Check sheet for the modelled part. Datum: model origin and axes. Units: mm. Face numbers are marked on the shaded views. Coordinates: 2 decimals unless noted, no trailing zeros. Answer as CSV lines item,"result". Start each with the question number.
1) Material ranges on L1, parallel to X at y = -4, z = 5.5; L2, parallel to X at y = -12, z = 3.5; L3, parallel to X at y = 8.5, z = 1.75, recorded low to high. Write a range as [from, to].
2) Section check A-A (z = 5.75). State how many separate pieces and enclosed holes the cut face has, and give its area (3 significant figures).
3) Draft check along X on the marked faces 1, 2 and 3. Enter one of: +X half, -X half, draft (parallel to the pull), parting line (faces both ways), or undercut.
4) Go/stop test with flat-tipped pins: pin 1 Ø3 at (x, y) = (0, -21) entering from +Z; pin 2 Ø4.5 at (x, y) = (0, 21) entering from -Z; pin 3 Ø1.5 at (y, z) = (-12, 2.5) entering from +X; pin 4 Ø1 at (x, z) = (-8.5, 2.5) entering from -Y. Record where each tip stops, or that it passes through.
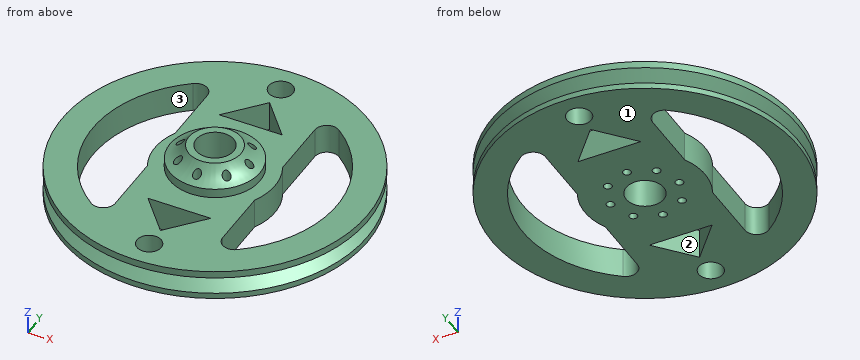
from build123d import *

# Parameters (mm, degrees)
F0_R      = 25.4
F0_R_2    = 3.125
F1_DEPTH  = 5
F2_R      = 7.5
F2_R_2    = 3.125
F3_DEPTH  = 4
F4_R      = 6.096
F6_R      = 2.020962
F7_DEPTH  = 5.001
F10_R     = 0.662213
F11_DEPTH = 9.001


with BuildPart() as f1:
    # F0 (on Top) → F1 (new body)
    with BuildSketch(Plane.XY):
        Circle(F0_R)
        with BuildLine():
            Line((-8.950036, 14.687379), (-8.950036, 4.46059))
            ThreePointArc((-8.950036, 4.46059), (-10, 0), (-8.950036, -4.46059))
            Line((-8.950036, -4.46059), (-8.950036, -14.687379))
            ThreePointArc((-8.950036, -14.687379), (-10.053051, -16.474953), (-12.145455, -16.290805))
            ThreePointArc((-12.145455, -16.290805), (-20.32, 0), (-12.145455, 16.290805))
            ThreePointArc((-12.145455, 16.290805), (-10.053051, 16.474953), (-8.950036, 14.687379))
        make_face(mode=Mode.SUBTRACT)
        Circle(F0_R_2, mode=Mode.SUBTRACT)
        with BuildLine():
            Line((8.950036, 4.46059), (8.950036, 14.687379))
            ThreePointArc((8.950036, 14.687379), (10.053051, 16.474953), (12.145455, 16.290805))
            ThreePointArc((12.145455, 16.290805), (20.32, 0), (12.145455, -16.290805))
            ThreePointArc((12.145455, -16.290805), (10.053051, -16.474953), (8.950036, -14.687379))
            Line((8.950036, -14.687379), (8.950036, -4.46059))
            ThreePointArc((8.950036, -4.46059), (10, 0), (8.950036, 4.46059))
        make_face(mode=Mode.SUBTRACT)
    extrude(amount=F1_DEPTH)

    # F2 (on face) → F3 (join)
    with BuildSketch(Plane.XY.offset(5)):
        Circle(F2_R)
        Circle(F2_R_2, mode=Mode.SUBTRACT)
    extrude(amount=F3_DEPTH)

    # F4 (on Front) → F5 (revolve, cut)
    with BuildSketch(Plane.XZ):
        with Locations((-9.469913, 12.312098)):
            Circle(F4_R)
    revolve(axis=Axis((0, 0, 5.050069), (0, 0, -1)), mode=Mode.SUBTRACT)

    # F6 (on face) → F7 (cut, through all)
    with BuildSketch(Plane.XY.offset(5)):
        Polygon((-5.234685, 11.362989), (0, 11.362989), (0, 17.41166), align=None)
        Polygon((0, 17.41166), (0, 11.362989), (5.234685, 11.362989), align=None)
        Polygon((0, -11.362989), (-5.234685, -11.362989), (0, -17.41166), (5.234685, -11.362989), align=None)
        with Locations((0, 20.997725)):
            Circle(F6_R)
        with Locations((0, -20.997725)):
            Circle(F6_R)
    extrude(amount=-F7_DEPTH, mode=Mode.SUBTRACT)

    # F8 (on Front) → F9 (revolve, cut)
    with BuildSketch(Plane.XZ):
        Polygon((-25.495, 3.902024), (-25.495, 2.402024), (-23.495, 2.402024), align=None)
        Polygon((-23.495, 2.402024), (-25.495, 2.402024), (-25.495, 0.902024), align=None)
    revolve(axis=Axis((0, 0, 20.538263), (0, 0, -1)), mode=Mode.SUBTRACT)

    # F10 (on face) → F11 (cut, through all)
    with BuildSketch(Plane.XY):
        with Locations((0, 5.743192)):
            Circle(F10_R)
        with Locations((-4.06105, 4.06105)):
            Circle(F10_R)
        with Locations((-5.743192, 0)):
            Circle(F10_R)
        with Locations((-4.06105, -4.06105)):
            Circle(F10_R)
        with Locations((0, -5.743192)):
            Circle(F10_R)
        with Locations((4.06105, -4.06105)):
            Circle(F10_R)
        with Locations((5.743192, 0)):
            Circle(F10_R)
        with Locations((4.06105, 4.06105)):
            Circle(F10_R)
    extrude(amount=F11_DEPTH, mode=Mode.SUBTRACT)


solid = f1.part
Results found:
1,L1,"x = [-6.34, -4.72], [-3.4, 3.4], [4.72, 6.34]"
1,L2,"x = [-21.88, -16.4], [-8.95, -4.68], [4.68, 8.95], [16.4, 21.88]"
1,L3,"x = [-22.83, -18.46], [-8.95, 8.95], [18.46, 22.83]"
2,separate pieces,"1"
2,enclosed holes,"9"
2,area,"135 mm2"
3,face 1,"draft"
3,face 2,"undercut"
3,face 3,"undercut"
4,pin 1,"passes through"
4,pin 2,"stops at z = 0"
4,pin 3,"stops at x = 21.58"
4,pin 4,"stops at y = -22.78"
